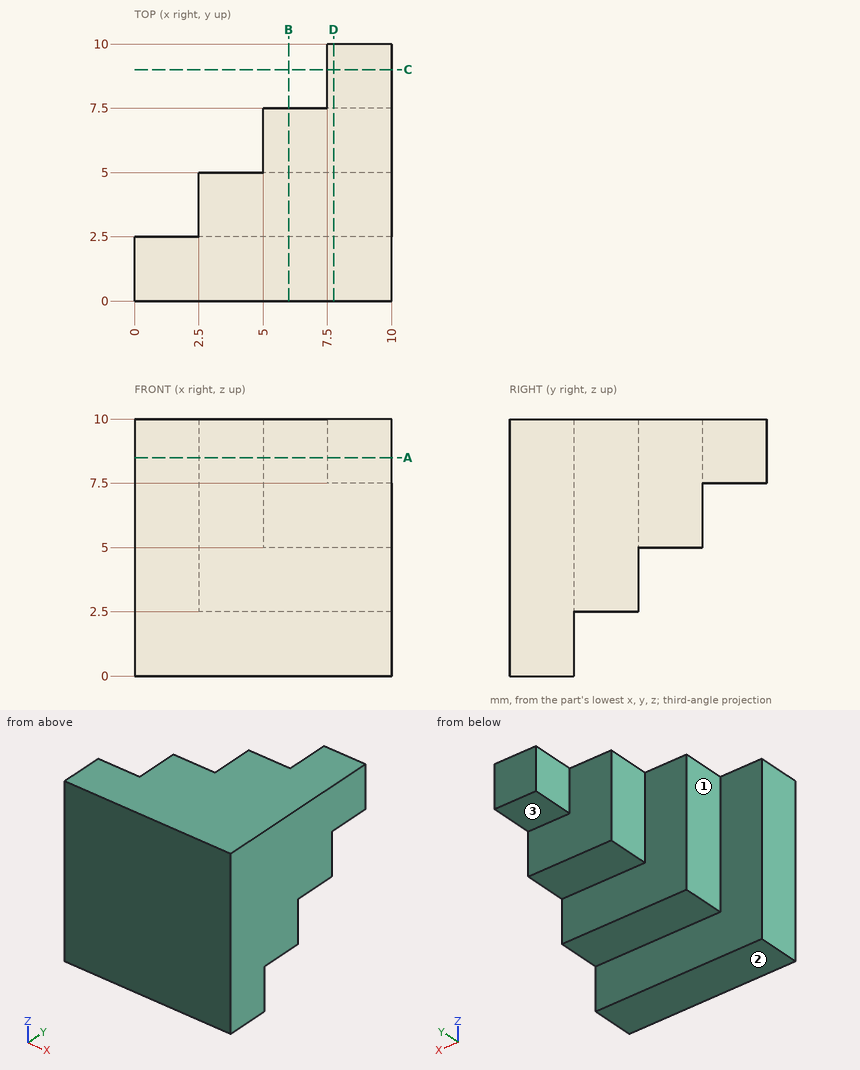
Verification items for this drawing (mm, ordinates from the low corner). A direction names the side the tool comes from. Coordinates: 2 decimals unless noted, no trailing zeros. Write each loop counter-clockwise with the first axis right and the second up, starting at its lowest first coordinate (ties: lowest second). Pieces come first, ordered by that corner, then holes. Notation, with made-up numbers: M -35.5,49 L 22.5,49 A14 ccw 22.5,69 Z; hole C 16,81.5 d11. An arc over 180 degrees is marked long. Answer as a JSON object with one key per item and string values.
1. Section check C-C, the plane y = 9. Enter the section's corners in (x, z), plus the area to 3 significant figures.
Answers below:
{"outline": "M 7.5,7.5 L 10,7.5 L 10,10 L 7.5,10 Z", "area": "6.25 mm²"}
2. Section check A-A, the plane z = 8.5. Enter the section's corners in (x, y), plus the area to 3 significant figures.
Answers below:
{"outline": "M 0,0 L 10,0 L 10,10 L 7.5,10 L 7.5,7.5 L 5,7.5 L 5,5 L 2.5,5 L 2.5,2.5 L 0,2.5 Z", "area": "62.5 mm²"}
3. Go/stop test with flat-tipped pins: pin 1 Ø0.8 at (y, z) = (9, 9) entering from -X; pin 2 Ø1.2 at (y, z) = (6.5, 8.5) entering from -X; pin 3 Ø4 at (x, z) = (6, 2.5) entering from +Y. Record where each tip stops, or that it passes through.
Answers below:
{"pin 1": "stops at x = 7.5", "pin 2": "stops at x = 5", "pin 3": "stops at y = 5"}
4. Tool access check on the marked faces 1, 2 and 3. Record the directions out of +Z, -Z, +X, -X, +Y, -Y that give a thin tool (end or side, any length) a straight path to the whole face; none if there is none.
Answers below:
{"face 1": "+Z, -Z, -X, +Y", "face 2": "-Z, +X, -X, +Y, -Y", "face 3": "-Z, +X, -X, +Y"}
5. Section check D-D, the plane x = 7.75. Enter the section's corners in (y, z), plus the area to 3 significant figures.
Answers below:
{"outline": "M 0,0 L 2.5,0 L 2.5,2.5 L 5,2.5 L 5,5 L 7.5,5 L 7.5,7.5 L 10,7.5 L 10,10 L 0,10 Z", "area": "62.5 mm²"}
6. Scan lines: L1, parallel to Y at x = 3, z = 9; L2, parallel to Z at x = 8.75, y = 7.25; L3, parallel to X at y = 7.75, z = 9.5. Record each from-to range of solid material in increasing order.
Answers below:
{"L1": "y = 0 to 5", "L2": "z = 5 to 10", "L3": "x = 7.5 to 10"}
7. Section check B-B, the plane x = 6. Enter the section's corners in (y, z), plus the area to 4 significant figures.
Answers below:
{"outline": "M 0,0 L 2.5,0 L 2.5,2.5 L 5,2.5 L 5,5 L 7.5,5 L 7.5,10 L 0,10 Z", "area": "56.25 mm²"}
